from build123d import *

# Parameters (mm, degrees)
BOSS_EXTRUDE1_DEPTH = 50
BOSS_EXTRUDE2_REACH = 113.636
SKETCH2_W           = 30
SKETCH2_H           = 14.135098559
SKETCH3_R           = 10
SKETCH3_R_2         = 5
BOSS_EXTRUDE3_DEPTH = 10
SKETCH4_R           = 15
CUT_EXTRUDE1_DEPTH  = 10
SKETCH5_W           = 10
SKETCH5_H           = 5
CUT_EXTRUDE2_DEPTH  = 123.622026278


with BuildPart() as part:
    # Sketch1 → Boss-Extrude1 (new body)
    with BuildSketch(Plane.XY):
        with BuildLine():
            Line((0, 0), (100, 0))
            Line((100, 0), (100, 30))
            Line((100, 30), (60, 30))
            Line((60, 30), (60, 25))
            ThreePointArc((60, 25), (57.071067812, 17.928932188), (50, 15))
            Line((50, 15), (0, 15))
            Line((0, 15), (0, 0))
        make_face()
    extrude(amount=-BOSS_EXTRUDE1_DEPTH)

    # Boss-Extrude2: up to this plane
    boss_extrude2_end = Plane(origin=(50, 15, -50), z_dir=(0, 1, 0))
    # Sketch2 → Boss-Extrude2 (add, up to the surface)
    with BuildSketch(Plane(origin=(7.5, -7.5, 0), x_dir=(0, 0, 1), z_dir=(-0.7071067811865489, 0.7071067811865462, 0)), mode=Mode.PRIVATE) as boss_extrude2_sk1:
        with Locations((-25, 38.894391498)):
            Rectangle(SKETCH2_W, SKETCH2_H)
    boss_extrude2_tool1 = split(extrude(boss_extrude2_sk1.sketch, amount=-BOSS_EXTRUDE2_REACH, mode=Mode.PRIVATE), bisect_by=boss_extrude2_end, keep=Keep.BOTH, mode=Mode.PRIVATE)
    add(boss_extrude2_tool1.solids().sort_by_distance((35.002488, 20.002488, -25))[0])
    # Sketch2 → Boss-Extrude2 (add, up to the surface)
    with BuildSketch(Plane(origin=(7.5, -7.5, 0), x_dir=(0, 0, 1), z_dir=(-0.7071067811865489, 0.7071067811865462, 0)), mode=Mode.PRIVATE) as boss_extrude2_sk2:
        with BuildLine():
            Line((-40, 61.826842218), (-40, 45.961940777))
            Line((-40, 45.961940777), (-10, 45.961940777))
            Line((-10, 45.961940777), (-10, 61.826842218))
            ThreePointArc((-10, 61.826842218), (-25, 76.826842218), (-40, 61.826842218))
        make_face()
    boss_extrude2_tool2 = split(extrude(boss_extrude2_sk2.sketch, amount=-BOSS_EXTRUDE2_REACH, mode=Mode.PRIVATE), bisect_by=boss_extrude2_end, keep=Keep.BOTH, mode=Mode.PRIVATE)
    add(boss_extrude2_tool2.solids().sort_by_distance((49.917636, 34.917636, -25))[0])

    # Sketch3 → Boss-Extrude3 (add)
    with BuildSketch(Plane(origin=(7.5, -7.5, 0), x_dir=(0, 0, 1), z_dir=(-0.7071067811865488, 0.7071067811865464, 0))):
        with Locations(Location((-25, 61.826842218, 0), (0, 0, 270))):
            Circle(SKETCH3_R)
        with Locations(Location((-25, 61.826842218, 0), (0, 0, 270))):
            Circle(SKETCH3_R_2, mode=Mode.SUBTRACT)
    extrude(amount=BOSS_EXTRUDE3_DEPTH)

    # Sketch4 → Cut-Extrude1 (cut)
    with BuildSketch(Plane(origin=(0, 30, 0), x_dir=(1, 0, 0), z_dir=(0, 1, 0))):
        with Locations((100, 50)):
            Circle(SKETCH4_R)
        with Locations((100, 0)):
            Circle(SKETCH4_R)
    extrude(amount=-CUT_EXTRUDE1_DEPTH, mode=Mode.SUBTRACT)

    # Sketch5 → Cut-Extrude2 (cut, through all)
    with BuildSketch(Plane.XY):
        with Locations((20, 2.5)):
            Rectangle(SKETCH5_W, SKETCH5_H)
        with Locations((80, 2.5)):
            Rectangle(SKETCH5_W, SKETCH5_H)
    extrude(amount=-CUT_EXTRUDE2_DEPTH, mode=Mode.SUBTRACT)


solid = part.part
Design review of the part built by this model. Coordinates are the model's own, in mm. A direction names the side the tool comes from. Round coordinates to 2 decimals unless told otherwise and drop trailing zeros. Write each loop counter-clockwise with the first axis right and the second up, starting at its lowest first coordinate (ties: lowest second). Pieces come first, ordered by that corner, then holes. Notation, with made-up numbers: M -11,34.5 L 16,34.5 A21 cw 16,39.5 Z; hole C 80,-1.5 d2. An arc over 180 degrees is marked long. One line per item, written item: value. Start each with the question number.
1. Take a section at A-A on x = 83.5. State the section outline as (y, z) points, then the cut area to 3 significant figures.
2. For faces 1 (the face through (94, 20, -44)), 2 (the face through (20, 5, -25)), 3 (the face through (20, 15, -25)), list the 3-axis set-ups (+Z, -Z, +X, -X, +Y, -Y) from which the entire face can be reached by the end or side of a thin tool; tool diameter is ignored.
3. Clearance check with flat-ended pins moving along their axes: P1, Ø25, axis at x = 24, z = -18.5, coming from the +Y side; P2, Ø16.5, axis at x = 91.5, z = -39, coming from the +Y side; P3, Ø1, axis at x = 57, z = -14.5, coming from the +Y side. State where each tip first meets the part, or that it passes through.
4. Take a section at D-D on z = -5. State the section outline as (x, y) points, then the cut area to 3 significant figures.
5. Take a section at B-B on z = -41.5. State the section outline as (x, y) points, then the cut area to 3 significant figures.
6. To check wall thickness, follow probe 1 along X at (y, z) = (4.5, -42.5); probe 2 along Y at (x, z) = (87, -37); probe 3 along Z at (x, y) = (53, 24). State the ranges of each line that lie inside material, in increasing order. Write a range as from..to.
Computed:
1. outline: M 5,-50 L 30,-50 L 30,0 L 5,0 Z
1. area: 1,250 mm²
2. face 1: -Z, +X, +Y
2. face 2: +Z, -Z, -Y
2. face 3: -X, +Y
3. P1: stops at y = 21.5
3. P2: stops at y = 30
3. P3: stops at y = 42.5
4. outline: M 0,0 L 15,0 L 15,5 L 25,5 L 25,0 L 75,0 L 75,5 L 85,5 L 85,0 L 100,0 L 100,20 L 85.86,20 L 85.86,30 L 60,30 L 60,25 A10 cw 50,15 L 0,15 Z
4. area: 1,880 mm²
5. outline: M 0,0 L 15,0 L 15,5 L 25,5 L 25,0 L 75,0 L 75,5 L 85,5 L 85,0 L 100,0 L 100,20 L 87.64,20 L 87.64,30 L 60,30 L 60,25 A10 cw 50,15 L 0,15 Z
5. area: 1,900 mm²
6. probe 1: x = 0..15, 25..75, 85..100
6. probe 2: y = 0..30
6. probe 3: z = -40..-10
